Source: CAD feature listing. Evaluate the final solid. Frame: model axes, mm. Face numbers are marked on the shaded views. A direction names the side the tool comes from. Round coordinates to 2 decimals unless told otherwise and drop trailing zeros. Order: outer loops, then holes, each group sorted by start corner. A loop starts at its lowest first (then second) coordinate and runs counter-clockwise, first axis right, second up. Notation, with made-up numbers: (3.25, 11.25) -> (23.25, 11.25) arc R26 cw to (23.25, 30.25) -> close; hole circle Ø2 at (60, 42.5). An arc over 180 degrees is marked (long way). One line per item, written item: value. Start each with the question number.
1) Section B-B (x = 1). Return the cut outline in (y, z).
2) Ray query, L1, parallel to Y at x = 4.5, z = 12.25; L2, parallel to X at y = 6, z = 7.75; L3, parallel to X at y = 6, z = -0.75. Return the intervals inside material, ascending.
3) Mould query, pull axis X, two halves, no side actions, for the marked faces 1, 2, 3 and 4. Classes: pulls with the +X half, pulls with the -X half, needs draft (parallel to the pull), parting line crosses it, or undercut.
4) Section A-A (y = 6.75). Return the cut outline in (x, z).
5) Section C-C (z = -0.75). Return the cut outline in (x, y), and give its area (3 significant figures).
6) Reachability of the marked faces 5 and 6 from +Z, -Z, +X, -X, +Y, -Y: full face, straight path, thin tool, end or side. Return the list, or none.
7) Pin query (flat end, axial travel): P1, Ø1.5, axis at x = 3, z = 9, coming from the +Y side. Return the tip coordinate at first contact, or that it passes through.
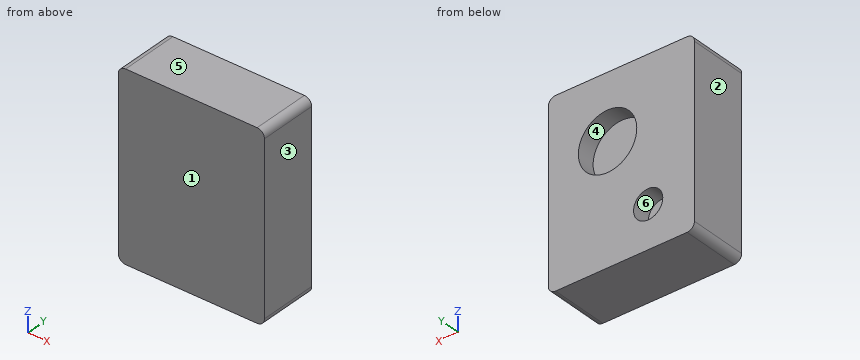
```python
from build123d import *

# Parameters (mm, degrees)
SKETCH1_W           = 20
SKETCH1_H           = 25
BOSS_EXTRUDE1_DEPTH = 8
FILLET1_R           = 1
SKETCH4_R           = 2
SKETCH4_R_2         = 4
CUT_EXTRUDE1_DEPTH  = 2.5


with BuildPart() as part:
    # Sketch1 → Boss-Extrude1 (new body)
    with BuildSketch(Plane(origin=(0, 0, 0), x_dir=(1, 0, 0), z_dir=(0, 1, 0))):
        with Locations((1.861702128, -5.053191489)):
            Rectangle(SKETCH1_W, SKETCH1_H)
    extrude(amount=BOSS_EXTRUDE1_DEPTH)

    # Fillet1
    fillet1_edges = [part.edges().sort_by_distance(p)[0] for p in [
        (-8.138297872, 4, -7.446808511),
        (-8.138297872, 4, 17.553191489),
        (11.861702128, 4, 17.553191489),
        (11.861702128, 4, -7.446808511),
    ]]
    fillet(fillet1_edges, radius=FILLET1_R)

    # Sketch4 → Cut-Extrude1 (cut)
    with BuildSketch(Plane(origin=(0, 8, 0), x_dir=(1, 0, 0), z_dir=(0, 1, 0))):
        with Locations(Location((-1.804003479, 1.636713319, 0), (0, 0, 270))):
            Circle(SKETCH4_R)
        with Locations(Location((3.755918293, -8.724959073, 0), (0, 0, 270))):
            Circle(SKETCH4_R_2)
    extrude(amount=-CUT_EXTRUDE1_DEPTH, mode=Mode.SUBTRACT)


solid = part.part
```
Findings:
1. outline: (0, -7.45) -> (8, -7.45) -> (8, 5.83) -> (5.5, 5.83) -> (5.5, 11.62) -> (8, 11.62) -> (8, 17.55) -> (0, 17.55) -> close
2. L1: 0 to 5.5
2. L2: -8.14 to -0.12, 7.64 to 11.86
2. L3: -8.14 to -3.6, -0.01 to 11.86
3. face 1: needs draft
3. face 2: pulls with the -X half
3. face 3: pulls with the +X half
3. face 4: undercut
4. outline: (-8.14, -6.45) arc R1 ccw to (-7.14, -7.45) -> (10.86, -7.45) arc R1 ccw to (11.86, -6.45) -> (11.86, 16.55) arc R1 ccw to (10.86, 17.55) -> (-7.14, 17.55) arc R1 ccw to (-8.14, 16.55) -> close; hole circle Ø4 at (-1.8, -1.64); hole circle Ø8 at (3.76, 8.72)
5. outline: (-8.14, 0) -> (11.86, 0) -> (11.86, 8) -> (-0.01, 8) -> (-0.01, 5.5) -> (-3.6, 5.5) -> (-3.6, 8) -> (-8.14, 8) -> close
5. area: 151 mm2
6. face 5: +Z, +X, -X, +Y, -Y
6. face 6: +Y
7. P1: y = 5.5
